Here's how the part is built. I have some questions about the finished solid (model axes, mm). Face numbers are marked on the shaded views. A direction names the side the tool comes from. Coordinates: 2 decimals unless noted, no trailing zeros. Order: outer loops, then holes, each group sorted by start corner. A loop starts at its lowest first (then second) coordinate and runs counter-clockwise, first axis right, second up. Notation, with made-up numbers: (9.25, -17.5) - (41.25, -17.5) arc R20 cw to (41.25, -4.5) - close; hole circle Ø6 at (11, 74.25). An arc over 180 degrees is marked (long way). Use one line per item in the form item = value. Start each with the question number.
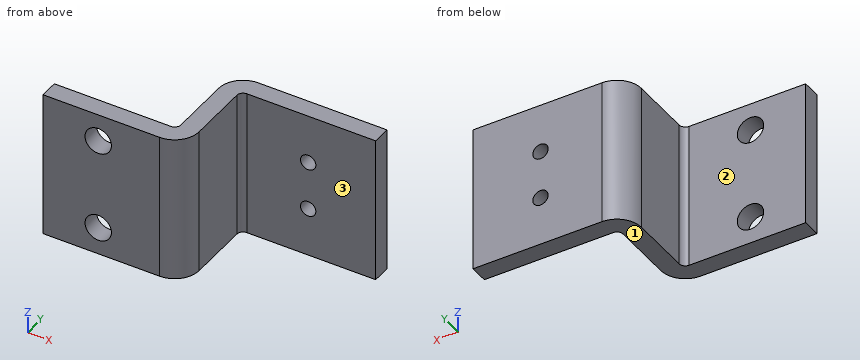
from build123d import *

# Parameters (mm, degrees)
SM_BASE_FLANGE_1_DEPTH = 24
HOLE_WIZARD_M4_1_D     = 4.3
M3X0_5_1_D             = 2.5


# Sheet-metal steps are written as plain solids
with BuildPart() as part:
    # Sketch 1 → 基材-凸緣1 (new body)
    with BuildSketch(Plane.XY):
        with BuildLine():
            Line((25, 15), (4, 15))
            ThreePointArc((4, 15), (1.171572875, 13.828427125), (0, 11))
            Line((0, 11), (0, 1))
            ThreePointArc((0, 1), (-0.292893219, 0.292893219), (-1, 0))
            Line((-1, 0), (-20, 0))
            Line((-20, 0), (-20, -3))
            Line((-20, -3), (-1, -3))
            ThreePointArc((-1, -3), (1.828427125, -1.828427125), (3, 1))
            Line((3, 1), (3, 11))
            ThreePointArc((3, 11), (3.292893219, 11.707106781), (4, 12))
            Line((4, 12), (25, 12))
            Line((25, 12), (25, 15))
        make_face()
    extrude(amount=SM_BASE_FLANGE_1_DEPTH)

    # M4 餘隙孔1 (through all)
    with Locations(Plane(origin=(0, 0, 0), x_dir=(1, 0, 0), z_dir=(0, 1, 0))):
        with Locations((-11, -19.5), (-11, -4.5)):
            Hole(HOLE_WIZARD_M4_1_D / 2)

    # M3x0.5 螺紋孔1 (through all)
    with Locations(Plane(origin=(0, 15, 0), x_dir=(1, 0, 0), z_dir=(0, 1, 0))):
        with Locations((14, -16), (14, -8)):
            Hole(M3X0_5_1_D / 2)


solid = part.part
1) For pin 1 (3 mm diameter, centred on x = 14, z = 8, fed in from -Y); pin 2 (2 mm diameter, centred on x = -9, z = 13, fed in from +Y); pin 3 (5 mm diameter, centred on y = 5, z = 15, fed in from -X); pin 4 (1 mm diameter, centred on x = -1, y = 10.5, fed in from -Z), each with a flat end and sliding along its axis, tell me the tip position at first contact or that it passes through.
2) Suppose I cut it at A-A, the plane x = 14. List the corners of the cut face in (y, z) for me.
3) Suppose I cut it at C-C, the plane z = 16. List the corners of the cut face in (x, y) for me.
4) Which directions (+Z, -Z, +X, -X, +Y, -Y) give clear straight access to the entire face, cutting with the end or side of a thin tool? Please do the marked faces 1, 2 and 3.
5) Suppose I cut it at B-B, the plane z = 19.5. List the corners of the cut face in (x, y) for me.
6) I need wall thicknesses on probe 1 along Z at (x, y) = (-11, -1.1); probe 2 along Z at (x, y) = (14, 13.65); probe 3 along Y at (x, z) = (-18, 12.5). Which ranges of each line are inside material? Lowest first, please. Write a range as [from, to].
7) Suppose I cut it at D-D, the plane y = 3.25. List the corners of the cut face in (x, z) for me, then the cut area to 3 significant figures.
From the geometry:
q1.pin_1 = 12
q1.pin_2 = 0
q1.pin_3 = 0
q1.pin_4 = through
q2.outline = (12, 0) - (15, 0) - (15, 6.75) - (12, 6.75) - close; (12, 9.25) - (15, 9.25) - (15, 14.75) - (12, 14.75) - close; (12, 17.25) - (15, 17.25) - (15, 24) - (12, 24) - close
q3.outline = (-20, -3) - (-1, -3) arc R4 ccw to (3, 1) - (3, 11) arc R1 cw to (4, 12) - (12.75, 12) - (12.75, 15) - (4, 15) arc R4 ccw to (0, 11) - (0, 1) arc R1 cw to (-1, 0) - (-20, 0) - close; (15.25, 12) - (25, 12) - (25, 15) - (15.25, 15) - close
q4.face_1 = -Z, +X, -X, +Y, -Y
q4.face_2 = +Z, -Z, -X, +Y
q4.face_3 = +Z, -Z, +X, -Y
q5.outline = (-20, -3) - (-13.15, -3) - (-13.15, 0) - (-20, 0) - close; (-8.85, -3) - (-1, -3) arc R4 ccw to (3, 1) - (3, 11) arc R1 cw to (4, 12) - (25, 12) - (25, 15) - (4, 15) arc R4 ccw to (0, 11) - (0, 1) arc R1 cw to (-1, 0) - (-8.85, 0) - close
q6.probe_1 = [0, 2.35], [6.65, 17.35], [21.65, 24]
q6.probe_2 = [0, 6.75], [9.25, 14.75], [17.25, 24]
q6.probe_3 = [-3, 0]
q7.outline = (0, 0) - (3, 0) - (3, 24) - (0, 24) - close
q7.area = 72.0 mm2
